Here's the drawing with two shaded views (mm, measured from the low corner). I have some questions. Give positions to 0.01 mm unless a question says otherwise; leave off trailing zeros. Write each loop counter-clockwise with the first axis right and the second up, starting at its lowest first coordinate (ties: lowest second). Pieces come first, ordered by that corner, then holes.
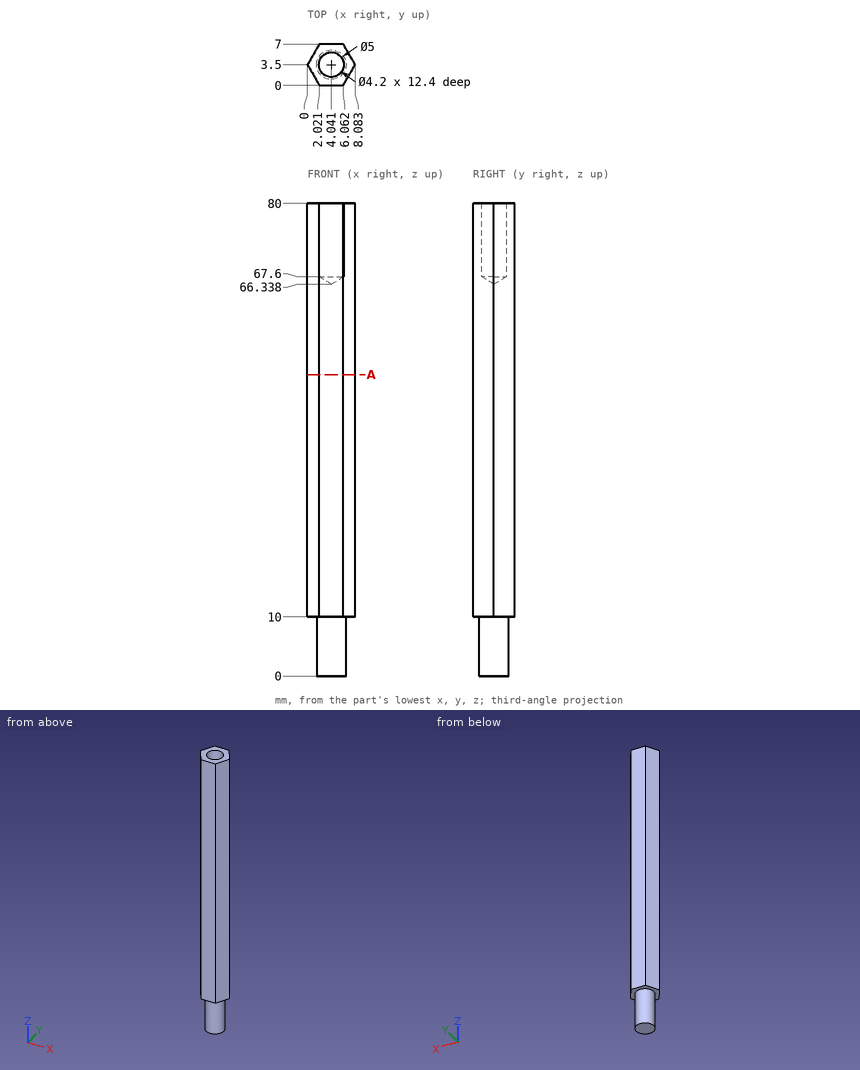
(1) Will these pins go through, and if not, where does the flat tip stop? P1, Ø1.5, axis at y = 1.5, z = 60.5, coming from the -X side; P2, Ø1.5, axis at y = 4.5, z = 51, coming from the -X side (1 decimal).
Returned:
P1: stops at x = 0.72
P2: stops at x = 0.1
(2) If I drill on L1, parallel to X at y = 3.5, z = 70; L2, parallel to Y at x = 4.25, z = 70; L3, parallel to Z at x = 1.5, y = 2.75, over which ranges is the centre line in solid material (lowest first)?
Returned:
L1: x = 0 to 1.94, 6.14 to 8.08
L2: y = 0 to 1.41, 5.59 to 7
L3: z = 10 to 80
(3) Imagine slicing it at A-A, the plane z = 51. Write out the boundary of the cut face in (x, y).
Returned:
outline: (0, 3.5) - (2.02, 0) - (6.06, 0) - (8.08, 3.5) - (6.06, 7) - (2.02, 7) - close
